Source: three-view drawing plus pictorial views. Frame: mm from the lowest corner of the part. Round coordinates to 2 decimals unless told otherwise and drop trailing zeros. Order: outer loops, then holes, each group sorted by start corner. A loop starts at its lowest first (then second) coordinate and runs counter-clockwise, first axis right, second up. Notation, with made-up numbers: (11, -3) - (58, -3) arc R30 cw to (58, 33) - close; hole circle Ø10 at (86.5, 27.5). An arc over 180 degrees is marked (long way). One line per item, written item: value. Start each with the question number.
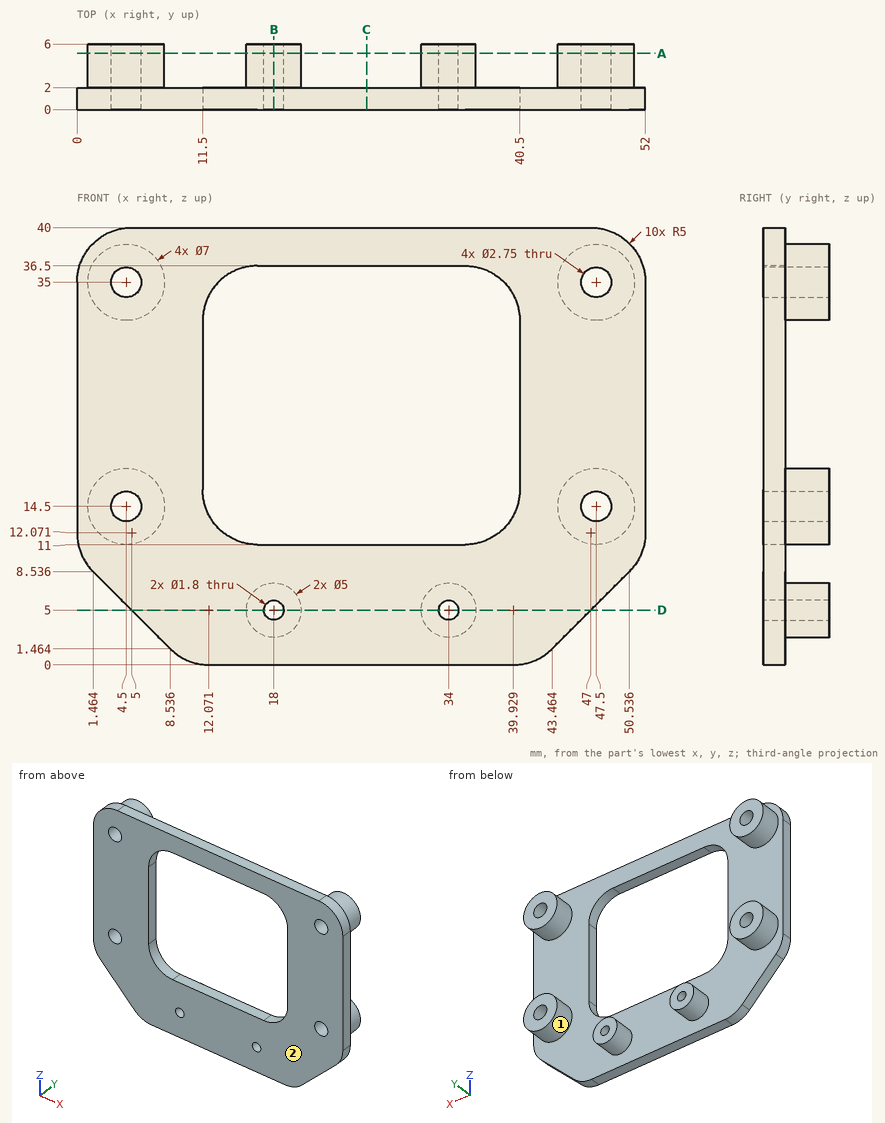
Item 1: Section query B-B on x = 18. Return loops of the section in (y, z).
Item 2: Line query: L1, parallel to X at y = 2.4, z = 5; L2, parallel to Z at x = 47.5, y = 4.75 (1 decimal); L3, parallel to X at y = 3.6, z = 35 (1 decimal). Output: solid intervals per line, ascending.
Item 3: Section query A-A on y = 5.15. Give the number of separate pieces and of enclosed holes in the cut face.
Item 4: Section query C-C on x = 26.5. Return loops of the section in (y, z).
Item 5: First-contact query: pin 1 Ø2 at (x, z) = (4.5, 35) entering from +Y; pin 2 Ø20 at (x, z) = (19.5, 29) entering from +Y; pin 3 Ø1 at (y, z) = (2, 7.5) entering from +X; pin 4 Ø3 at (y, z) = (3, 8.5) entering from -X. Flat tips, straight axial feed; report the tip coordinate or a pass-through.
Item 6: Pull-direction query (X, two-part tool) for the marked faces 1 and 2; classes: released by +X, released by -X, zero draft, split by the parting line, or undercut.
Item 7: Section query D-D on z = 5. Return loops of the section in (x, y).
Geometry results:
1. outline: (0, 0) - (2, 0) - (2, 2.5) - (6, 2.5) - (6, 4.1) - (0, 4.1) - close; (0, 5.9) - (6, 5.9) - (6, 7.5) - (2, 7.5) - (2, 11) - (0, 11) - close; (0, 36.5) - (2, 36.5) - (2, 40) - (0, 40) - close
2. L1: x = 15.5 to 17.1, 18.9 to 20.5, 31.5 to 33.1, 34.9 to 36.5
2. L2: z = 11 to 13.1, 15.9 to 18, 31.5 to 33.6, 36.4 to 38.5
2. L3: x = 1 to 3.1, 5.9 to 8, 44 to 46.1, 48.9 to 51
3. separate pieces: 6
3. enclosed holes: 6
4. outline: (0, 0) - (2, 0) - (2, 11) - (0, 11) - close; (0, 36.5) - (2, 36.5) - (2, 40) - (0, 40) - close
5. pin 1: passes through
5. pin 2: stops at y = 2
5. pin 3: stops at x = 50
5. pin 4: stops at x = 0.64
6. face 1: undercut
6. face 2: zero draft
7. outline: (5, 0) - (17.1, 0) - (17.1, 6) - (15.5, 6) - (15.5, 2) - (5, 2) - close; (18.9, 0) - (33.1, 0) - (33.1, 6) - (31.5, 6) - (31.5, 2) - (20.5, 2) - (20.5, 6) - (18.9, 6) - close; (34.9, 0) - (47, 0) - (47, 2) - (36.5, 2) - (36.5, 6) - (34.9, 6) - close
